from build123d import *

# Parameters (mm, degrees)
F0_R     = 4.55
F0_R_2   = 1.25
F1_DEPTH = 8
F2_SIZE2 = 2.5
F2_SIZE  = 5
F3_R     = 4.55
F3_R_2   = 3.25
F3_R_3   = 2.075
F3_R_4   = 1.25
F4_DEPTH = 2


with BuildPart() as f1:
    # F0 (on Top) → F1 (new body)
    with BuildSketch(Plane.XY):
        Circle(F0_R)
        Circle(F0_R_2, mode=Mode.SUBTRACT)
    extrude(amount=F1_DEPTH)

    # F2
    f2_edges = [f1.edges().sort_by_distance(p)[0] for p in [
        (-1.25, 0, 8),
    ]]
    f2_side = f1.faces().sort_by_distance((-1.25, 0, 4))[0]
    chamfer(f2_edges, length=F2_SIZE, length2=F2_SIZE2, reference=f2_side)

    # F3 (on face) → F4 (cut)
    with BuildSketch(Plane(origin=(0, 0, 0), x_dir=(1, 0, 0), z_dir=(0, 0, -1))):
        Circle(F3_R)
        Circle(F3_R_2, mode=Mode.SUBTRACT)
        Circle(F3_R_3)
        Circle(F3_R_4, mode=Mode.SUBTRACT)
    extrude(amount=-F4_DEPTH, mode=Mode.SUBTRACT)


solid = f1.part
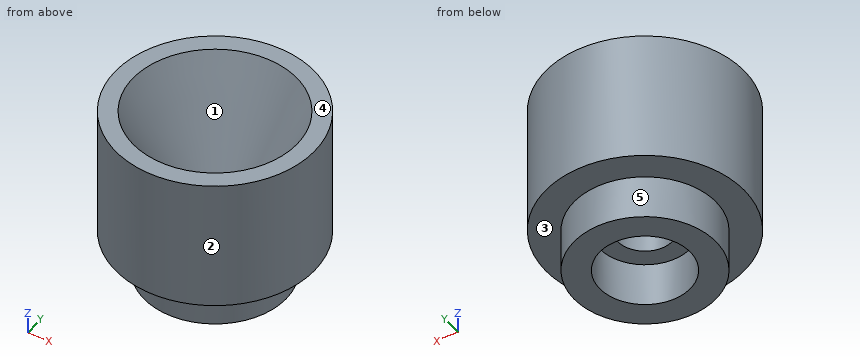
Model file for the job. Use its own axes, mm. Face numbers are marked on the shaded views. A direction names the side the tool comes from. Coordinates: 2 decimals unless noted, no trailing zeros. Write each loop counter-clockwise with the first axis right and the second up, starting at its lowest first coordinate (ties: lowest second). Pieces come first, ordered by that corner, then holes. Notation, with made-up numbers: (-37.75, -25) - (15.25, -25) arc R21 ccw to (15.25, -1) - close; hole circle Ø6 at (56.25, 38.25). An arc over 180 degrees is marked (long way). Write each question's results on one line, items separated by ' | '. Start each with the question number.
1) Cut at A-A (x = 0). Write the cut outline in (y, z) (3 decimals).
2) Cut at C-C (z = 0.5). Write the cut outline in (x, y) (3 decimals), then the cut area to 3 significant figures.
3) 3-axis set-ups, long thin cutter, end or side, ignore diameter. For the marked faces 4 and 5: which of +Z, -Z, +X, -X, +Y, -Y reach the whole face in a straight line?
4) Probe line 1 along Y through (x, z) = (0, 0.9) (3 decimals); line 2 along Y through (x, z) = (0, 2.7). List the from-to ranges inside material, lowest first. Write a range as from..to.
5) Flat gauge pins, fed straight in: P1, Ø2, axis at x = -3, z = 6.5, coming from the -Y side; P2, Ø2, axis at x = 3.5, z = 3, coming from the +Y side; P3, Ø1.2, axis at x = 1, y = 0.5, coming from the -Z side; P4, Ø2, axis at x = 0, y = 0, coming from the +Z side. Where does each tip first touch, or does it go through?
6) Cut at D-D (z = 2.5). Write the cut outline in (x, y).
7) Mould opens along X. For the marked faces 1, 2 and 3 say: pulls with the +X half, pulls with the -X half, needs draft (parallel to the pull), parting line crosses it, or undercut.
Returned:
1) outline: (-4.55, 2) - (-3.25, 2) - (-3.25, 0) - (-2.075, 0) - (-2.075, 2) - (-1.25, 2) - (-1.25, 3) - (-3.75, 8) - (-4.55, 8) - close; (1.25, 2) - (2.075, 2) - (2.075, 0) - (3.25, 0) - (3.25, 2) - (4.55, 2) - (4.55, 8) - (3.75, 8) - (1.25, 3) - close
2) outline: circle Ø6.5 at (0, 0); hole circle Ø4.15 at (0, 0) | area: 19.7 mm^2
3) face 4: +Z, +X, -X, +Y, -Y | face 5: -Z
4) line 1: -3.25..-2.075, 2.075..3.25 | line 2: -4.55..-1.25, 1.25..4.55
5) P1: y = -4.09 | P2: y = 3.8 | P3: z = 2 | P4: through
6) outline: circle Ø9.1 at (0, 0); hole circle Ø2.5 at (0, 0)
7) face 1: undercut | face 2: parting line crosses it | face 3: needs draft
